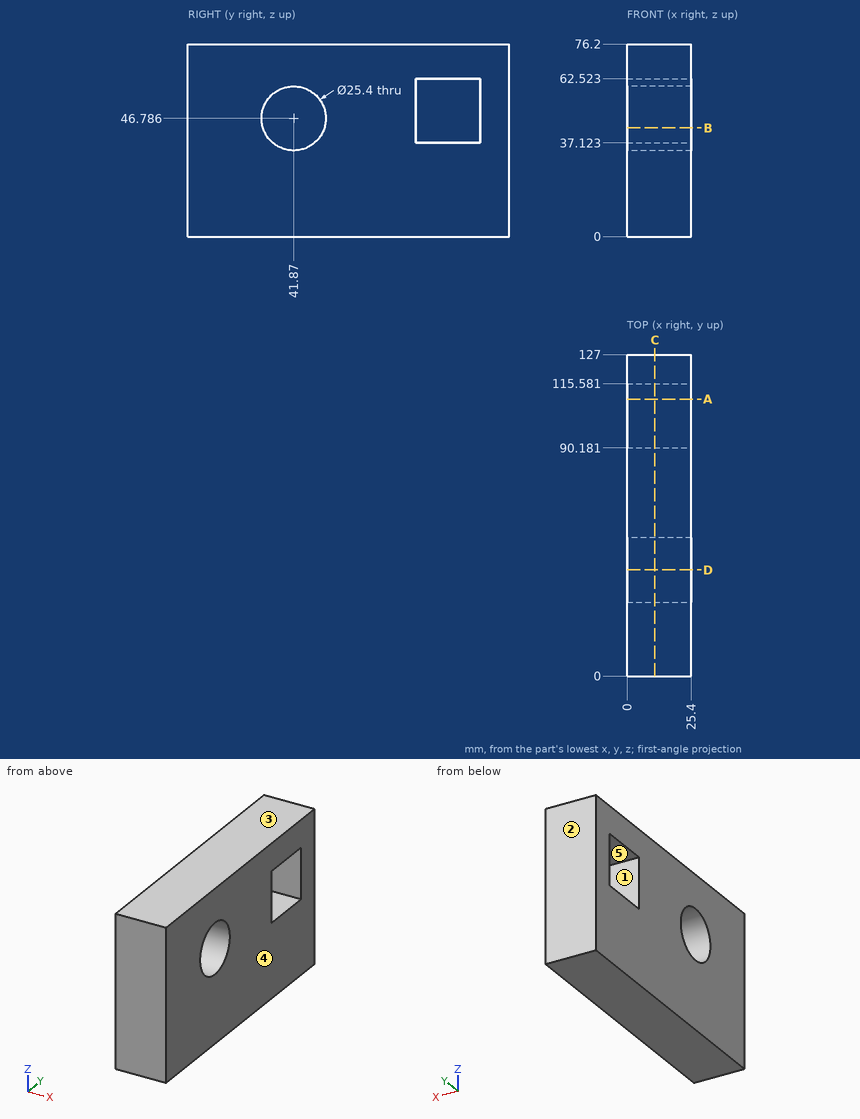
Study the drawing (mm; zero at the part's minimum x, y, z) and answer. A direction names the side the tool comes from. Round coordinates to 2 decimals unless told otherwise and drop trailing zeros. Order: outer loops, then holes, each group sorted by start corner. A loop starts at its lowest first (then second) coordinate and runs counter-clockwise, first axis right, second up. Notation, with made-up numbers: (56, -16.75) - (85, -16.75) arc R30 cw to (85, 8.25) - close; hole circle Ø11 at (84, 33). An arc over 180 degrees is marked (long way). Use one line per item in the form item = value. Start each with the question number.
(1) The part is cut by section C-C (x = 11). Give the vertices of the cut face in (y, z) (1 decimal).
(2) For the marked faces 1 and 2, determine the directions among +Z, -Z, +X, -X, +Y, -Y from which every point of the face is accessible in a straight line to the end or side of a thin tool.
(3) Find the intervals of material crossed by line 1 along Y through (x, z) = (23.5, 46) (1 decimal); line 2 along Z through (x, y) = (18.5, 110); line 3 along Y through (x, z) = (23, 42) (1 decimal), in increasing order. Write a range as from..to.
(4) The part is cut by section A-A (y = 109.5). Give the vertices of the cut face in (x, z).
(5) Determine the mould class of the marked faces 3, 4 and 5 for opening direction Z: +Z half, -Z half, draft (parallel to the pull), parting line (faces both ways), or undercut.
(6) The part is cut by section B-B (z = 43). Give the vertices of the cut face in (x, y).
(7) The part is cut by section D-D (y = 42). Give the vertices of the cut face in (x, z) (1 decimal).
Checked values:
q1.outline = (0, 0) - (127, 0) - (127, 76.2) - (0, 76.2) - close; hole circle Ø25.4 at (41.9, 46.8); hole (90.2, 37.1) - (115.6, 37.1) - (115.6, 62.5) - (90.2, 62.5) - close
q2.face_1 = +X, -X
q2.face_2 = +Z, -Z, +X, -X, +Y
q3.line_1 = 0..29.2, 54.5..90.2, 115.6..127
q3.line_2 = 0..37.12, 62.52..76.2
q3.line_3 = 0..30.1, 53.6..90.2, 115.6..127
q4.outline = (0, 0) - (25.4, 0) - (25.4, 37.12) - (0, 37.12) - close; (0, 62.52) - (25.4, 62.52) - (25.4, 76.2) - (0, 76.2) - close
q5.face_3 = +Z half
q5.face_4 = draft
q5.face_5 = undercut
q6.outline = (0, 0) - (25.4, 0) - (25.4, 29.75) - (0, 29.75) - close; (0, 53.99) - (25.4, 53.99) - (25.4, 90.18) - (0, 90.18) - close; (0, 115.58) - (25.4, 115.58) - (25.4, 127) - (0, 127) - close
q7.outline = (0, 0) - (25.4, 0) - (25.4, 34.1) - (0, 34.1) - close; (0, 59.5) - (25.4, 59.5) - (25.4, 76.2) - (0, 76.2) - close
